Here's how the part is built. I have some questions about the finished solid (model axes, mm). Face numbers are marked on the shaded views. A direction names the side the tool comes from. Coordinates: 2 decimals unless noted, no trailing zeros. Write each question's results on one line, items separated by ' | '. Start each with the question number.
from build123d import *

# Parameters (mm, degrees)
CYLINDER_R     = 7
CYLINDER_DEPTH = 5
SKETCH_W       = 5.4
SKETCH_H       = 3.6
SKETCH_W_2     = 3
SKETCH_H_2     = 1.2
PAD_DEPTH      = 15.5


with BuildPart() as cylinder:
    # Cylinder → Cylinder (new body)
    with BuildSketch(Plane.XY.offset(12.8)):
        Circle(CYLINDER_R)
    extrude(amount=CYLINDER_DEPTH)


with BuildPart() as body001:
    # Sketch001 → Revolution (revolve)
    with BuildSketch(Plane.XZ):
        with BuildLine():
            ThreePointArc((0, 15.8), (-7.9, 13.683201), (-13.683201, 7.9))
            Line((-10.392305, 6), (-13.683201, 7.9))
            ThreePointArc((0, 12), (-6, 10.392305), (-10.392305, 6))
            Line((0, 15.8), (0, 12))
        make_face()
    revolve(axis=Axis((0, 0, 0), (0, 0, 1)))


with BuildPart() as cut:
    # Sketch → Pad (new body)
    with BuildSketch(Plane.XY):
        Rectangle(SKETCH_W, SKETCH_H)
        Rectangle(SKETCH_W_2, SKETCH_H_2, mode=Mode.SUBTRACT)
    extrude(amount=PAD_DEPTH)

    # Boolean: union Body001
    add(body001.part)

    # Cut: cut Cylinder
    add(cylinder.part, mode=Mode.SUBTRACT)


solid = cut.part
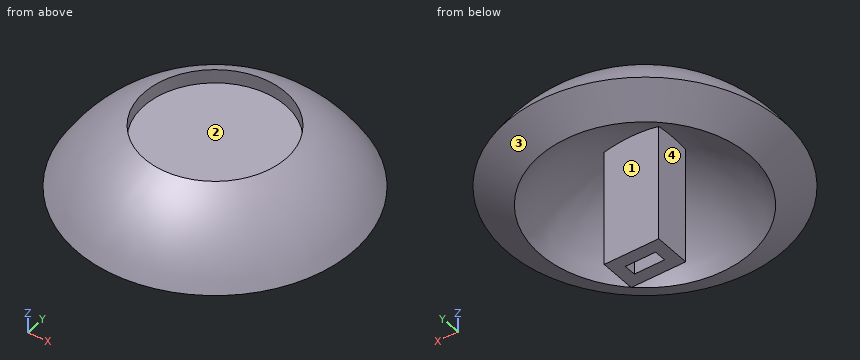
1) I want a section at A-A, the plane z = 10. Give the number of separate pieces and of enclosed holes in the cut face, then the cut area to 3 significant figures.
2) For the marked faces 1 and 2, which set-ups out of +Z, -Z, +X, -X, +Y, -Y let a thin tool reach every point of the face, with its end or its side?
3) We'd pull the mould along X, two halves only. Please class the marked faces 3 and 4: pulls with the +X half, pulls with the -X half, needs draft (parallel to the pull), parting line crosses it, or undercut.
4) For pin 1 Ø2.5 at (x, z) = (0, 6) entering from -Y; pin 2 Ø4 at (y, z) = (4, 11) entering from +X; pin 3 Ø3.5 at (x, z) = (-0.5, 4) entering from +Y, each with a flat end and sliding along its axis, tell me the tip position at first contact or that it passes through.
5) Please list where these lines run through material, in increasing order: line 1 (X direction, y = 0.25, z = 1); line 2 (Y direction, x = 1.75, z = 8.5); line 3 (X direction, y = 0, z = 10.5). Write a range as [from, to].
Output:
1) separate pieces: 2 | enclosed holes: 2 | area: 348 mm2
2) face 1: -Z | face 2: +Z
3) face 3: parting line crosses it | face 4: undercut
4) pin 1: stops at y = -12.56 | pin 2: stops at x = 12.47 | pin 3: stops at y = 1.8
5) line 1: x = [-2.7, -1.5], [1.5, 2.7] | line 2: y = [-13.2, -8.29], [-1.8, 1.8], [8.29, 13.2] | line 3: x = [-11.81, -5.81], [-2.7, -1.5], [1.5, 2.7], [5.81, 11.81]
